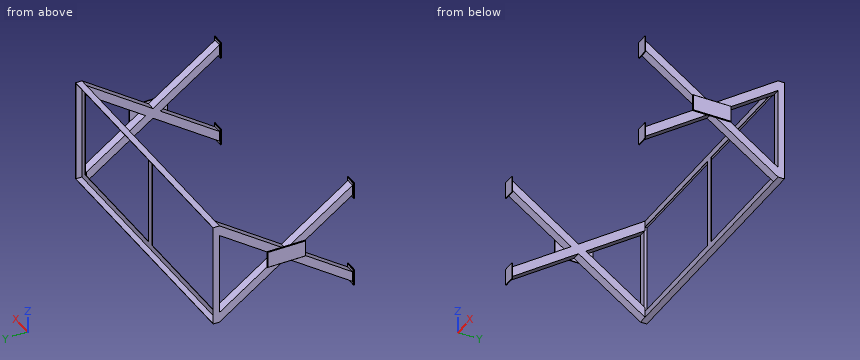
from build123d import *

# Parameters (mm, degrees)
CROQUIS1_W                 = 1540
CROQUIS1_H                 = 620
SALIENTE_EXTRUIR1_DEPTH    = 38.1
VACIADO1_T                 = -2
CROQUIS2_W                 = 1463.8
CROQUIS2_H                 = 543.8
CORTAR_EXTRUIR1_DEPTH      = 38.1
SALIENTE_EXTRUIR2_DEPTH    = 50.8
CROQUIS4_W                 = 100
CROQUIS4_H                 = 230
SALIENTE_EXTRUIR3_DEPTH    = 6
CHAFL_N1_SIZE              = 2
CROQUIS5_W                 = 70
CROQUIS5_H                 = 100
SALIENTE_EXTRUIR4_DEPTH    = 6
CHAFL_N2_SIZE              = 2
CHAFL_N2_OF_SIMETR_A2_SIZE = 2
CROQUIS6_W                 = 38.1
CROQUIS6_H                 = 543.8
SALIENTE_EXTRUIR5_DEPTH    = 2


# Read off the part's stored shape, not the designer's step: Simetría3
with BuildPart() as part:
    # Croquis1 → Saliente-Extruir1 (new body)
    with BuildSketch(Plane(origin=(0, 0, 0), x_dir=(1, 0, 0), z_dir=(0, 1, 0))):
        Rectangle(CROQUIS1_W, CROQUIS1_H)
    extrude(amount=SALIENTE_EXTRUIR1_DEPTH)

    # Vaciado1
    vaciado1_openings = [part.faces().sort_by_distance(p)[0] for p in [
        (0, 38.1, 0),
    ]]
    offset(amount=VACIADO1_T, openings=vaciado1_openings, kind=Kind.INTERSECTION)

    # Croquis2 → Cortar-Extruir1 (cut)
    with BuildSketch(Plane(origin=(0, 2, 0), x_dir=(1, 0, 0), z_dir=(0, 1, 0))):
        Rectangle(CROQUIS2_W, CROQUIS2_H)
    extrude(amount=-CORTAR_EXTRUIR1_DEPTH, mode=Mode.SUBTRACT)

    # Croquis3 → Saliente-Extruir2 (add)
    with BuildSketch(Plane(origin=(770, 0, 0), x_dir=(0, 0, -1), z_dir=(1, 0, 0))):
        Polygon((-310, 0), (-30.946230524, -400.95), (-310, -801.9), (-248.107538953, -801.9), (0, -445.414158831), (248.107538953, -801.9), (310, -801.9), (30.946230524, -400.95), (310, 0), (248.107538953, 0), (0, -356.485841169), (-248.107538953, 0), align=None)
    extrude(amount=-SALIENTE_EXTRUIR2_DEPTH)

    # Croquis4 → Saliente-Extruir3 (add)
    with BuildSketch(Plane(origin=(770, 0, 0), x_dir=(0, 0, -1), z_dir=(1, 0, 0))):
        with Locations((0, -400.95)):
            Rectangle(CROQUIS4_W, CROQUIS4_H)
    extrude(amount=SALIENTE_EXTRUIR3_DEPTH)

    # Chaflán1
    chafl_n1_edges = [part.edges().sort_by_distance(p)[0] for p in [
        (776, -400.95, -50),
        (776, -285.95, 0),
        (776, -400.95, 50),
        (776, -515.95, 0),
    ]]
    chamfer(chafl_n1_edges, length=CHAFL_N1_SIZE)

    # Croquis5 → Saliente-Extruir4 (add)
    with BuildSketch(Plane.XZ.offset(801.9)):
        with Locations((744.6, 279.053769476)):
            Rectangle(CROQUIS5_W, CROQUIS5_H)
    saliente_extruir4 = extrude(amount=SALIENTE_EXTRUIR4_DEPTH)

    # Chaflán2
    chafl_n2_edges = [part.edges().sort_by_distance(p)[0] for p in [
        (779.6, -801.9, 279.053769476),
        (744.6, -801.9, 329.053769476),
        (709.6, -801.9, 279.053769476),
        (744.6, -801.9, 229.053769476),
    ]]
    chamfer(chafl_n2_edges, length=CHAFL_N2_SIZE)

    # Simetría2: Saliente-Extruir4 across plane
    add(saliente_extruir4.mirror(Plane.XY))

    # Chaflán2 of Simetría2
    chafl_n2_of_simetr_a2_edges = [part.edges().sort_by_distance(p)[0] for p in [
        (779.6, -801.9, -279.053769476),
        (744.6, -801.9, -329.053769476),
        (709.6, -801.9, -279.053769476),
        (744.6, -801.9, -229.053769476),
    ]]
    chamfer(chafl_n2_of_simetr_a2_edges, length=CHAFL_N2_OF_SIMETR_A2_SIZE)

    # Croquis6 → Saliente-Extruir5 (add)
    with BuildSketch(Plane.XZ):
        Rectangle(CROQUIS6_W, CROQUIS6_H)
    extrude(amount=-SALIENTE_EXTRUIR5_DEPTH)

    # Simetría3: part across plane


with BuildPart() as part_1:
    add(part.part)
    add(part.part.mirror(Plane(origin=(0, 0, 0), x_dir=(0, 0, 1), z_dir=(1, 0, 0))))


solid = part_1.part
The model under review builds one solid part; all positions refer to its coordinate system, in mm. Round coordinates to 2 decimals unless told otherwise and drop trailing zeros. Write each loop counter-clockwise with the first axis right and the second up, starting at its lowest first coordinate (ties: lowest second). Pieces come first, ordered by that corner, then holes. Notation, with made-up numbers: (-25, -26) - (-9, -26) arc R21 cw to (-9, -12) - close; hole circle Ø10 at (30.5, -13.5). An arc over 180 degrees is marked (long way). One line per item, written item: value. Start each with the question number.
1. Clearance check with flat-ended pins moving along their axes: P1, Ø15, axis at y = -413.5, z = -37.5, coming from the +X side; P2, Ø2, axis at x = -772, y = -398.5, coming from the -Z side; P3, Ø15, axis at y = -396, z = 45, coming from the -X side. State where each tip first meets the part, or that it passes through.
2. Consider section A-A on x = 541. Write out the cut boundary in (y, z), and give its area (3 significant figures).
3. To check wall thickness, follow L1, parallel to X at y = -765, z = -275; L2, parallel to Y at x = -491, z = -300.5; L3, parallel to X at y = -307.5, z = -22. State the ranges of each line that lie inside material, in increasing order. Write a range as from..to.
4. Consider section C-C on y = -262.5. Write out the cut boundary in (x, z), and give its area (3 significant figures).
5. Consider section B-B on z = 145.5. State how many separate pieces and enclosed holes the cut face has, and give its area (3 significant figures).
Checks:
1. P1: stops at x = 776
1. P2: stops at z = -50
1. P3: stops at x = -776
2. outline: (0, -310) - (38.1, -310) - (38.1, -308) - (2, -308) - (2, -271.9) - (0, -271.9) - close; (0, 271.9) - (2, 271.9) - (2, 308) - (38.1, 308) - (38.1, 310) - (0, 310) - close
2. area: 297 mm^2
3. L1: x = -770..-719.2, 719.2..770
3. L2: y = 0..2
3. L3: x = -776..-770, 770..776
4. outline: (-770, -127.3) - (-719.2, -127.3) - (-719.2, -65.41) - (-770, -65.41) - close; (-770, 65.41) - (-719.2, 65.41) - (-719.2, 127.3) - (-770, 127.3) - close; (719.2, -127.3) - (770, -127.3) - (770, -65.41) - (719.2, -65.41) - close; (719.2, 65.41) - (770, 65.41) - (770, 127.3) - (719.2, 127.3) - close
4. area: 12,600 mm^2
5. separate pieces: 7
5. enclosed holes: 0
5. area: 18,400 mm^2
